from build123d import *

# Parameters (mm, degrees)
ESQUISSE2_R                                       = 76.2
ESQUISSE2_R_2                                     = 50.8
BOSS_EXTRU_1_DEPTH                                = 10
CHANFREIN1_SIZE                                   = 3
D_GAGEMENT_81_D                                   = 4.4958
FRAISAGE_POUR_VIS_T_TE_FRAIS_E_BOMB_E_D           = 5.1054
FRAISAGE_POUR_VIS_T_TE_FRAIS_E_BOMB_E_CSINK_D     = 9.779
FRAISAGE_POUR_VIS_T_TE_FRAIS_E_BOMB_E_CSINK_ANGLE = 82


with BuildPart() as part:
    # Esquisse2 → Boss.-Extru.1 (new body)
    with BuildSketch(Plane.XY):
        Circle(ESQUISSE2_R)
        Circle(ESQUISSE2_R_2, mode=Mode.SUBTRACT)
    extrude(amount=BOSS_EXTRU_1_DEPTH)

    # Chanfrein1
    chanfrein1_edges = [part.edges().sort_by_distance(p)[0] for p in [
        (-76.2, 0, 0),
    ]]
    chamfer(chanfrein1_edges, length=CHANFREIN1_SIZE)

    # Dégagement #81 (through all)
    with Locations(Plane(origin=(0, 0, 0), x_dir=(-1, 0, 0), z_dir=(0, 0, -1))):
        with Locations((0, 59.65), (51.658415336, 29.825), (29.825, 51.658415336), (59.65, 0), (51.658415336, -29.825), (29.825, -51.658415336), (0, -59.65), (-29.825, -51.658415336), (-51.658415336, -29.825), (-59.65, 0), (-51.658415336, 29.825), (-29.825, 51.658415336)):
            Hole(D_GAGEMENT_81_D / 2)

    # Fraisage pour vis à tête fraisée bombée #101 (through all)
    with Locations(Plane(origin=(0, 0, 0), x_dir=(-1, 0, 0), z_dir=(0, 0, -1))):
        with Locations((48.083261121, -48.083261121), (-65.682956188, -17.599695067), (17.599695067, 65.682956188)):
            CounterSinkHole(FRAISAGE_POUR_VIS_T_TE_FRAIS_E_BOMB_E_D / 2, FRAISAGE_POUR_VIS_T_TE_FRAIS_E_BOMB_E_CSINK_D / 2, counter_sink_angle=FRAISAGE_POUR_VIS_T_TE_FRAIS_E_BOMB_E_CSINK_ANGLE)


solid = part.part
The model under review builds one solid part; all positions refer to its coordinate system, in mm. Coordinates: 2 decimals unless noted, no trailing zeros. Write each loop counter-clockwise with the first axis right and the second up, starting at its lowest first coordinate (ties: lowest second). Pieces come first, ordered by that corner, then holes. Notation, with made-up numbers: (54.25, -6.5) - (87.25, -6.5) arc R23 cw to (87.25, 1.5) - close; hole circle Ø8 at (-38, 26). An arc over 180 degrees is marked (long way). Answer as CSV lines item,"result".
(1) Mouldability with a two-part tool opening along X and no side actions: class faces 1 (the conical face through (-45.62, -49.1, 2.56)), 2 (the flat face through (-52, 1, 10)), 3 (the conical face through (69.959, 22.031, 0.146)) as pulls with the +X half, pulls with the -X half, needs draft (parallel to the pull), parting line crosses it, or undercut.
Data:
face 1,"undercut"
face 2,"needs draft"
face 3,"parting line crosses it"
(2) Clearance check with flat-ended pins moving along their axes: pin 1 Ø1.5 at (x, z) = (7.5, 5) entering from -Y; pin 2 Ø4 at (y, z) = (36.5, 7.5) entering from -X; pin 3 Ø6 at (y, z) = (23.5, 5.5) entering from -X. State where each tip first meets the part, or that it passes through.
Data:
pin 1,"stops at y = -75.9"
pin 2,"stops at x = -67.94"
pin 3,"stops at x = -73.39"
(3) We need section A-A (y = 0). Give the boundary of the cut face in (x, z), plus the area to 3 significant figures.
Data:
outline,"(-76.2, 3) - (-73.2, 0) - (-61.9, 0) - (-61.9, 10) - (-76.2, 10) - close; (-57.4, 0) - (-50.8, 0) - (-50.8, 10) - (-57.4, 10) - close; (50.8, 0) - (57.4, 0) - (57.4, 10) - (50.8, 10) - close; (61.9, 0) - (73.2, 0) - (76.2, 3) - (76.2, 10) - (61.9, 10) - close"
area,"409 mm2"
(4) We need section C-C (z = 6.75). Count the separate pieces of the cut face and the enclosed holes in it, plus the area to 3 significant figures.
Data:
separate pieces,"1"
enclosed holes,"16"
area,"9,880 mm2"
(5) For line 1 along Y through (x, z) = (0, 6); line 2 along Y through (x, z) = (29, 6); line 3 along X through (y, z) = (11, 8.75), list the stretches that pass through material, from the lowest coordinate up. Write a range as [from, to].
Data:
line 1,"y = [-76.2, -61.9], [-57.4, -50.8], [50.8, 57.4], [61.9, 76.2]"
line 2,"y = [-70.47, -53.75], [-49.57, -41.71], [41.71, 49.57], [53.75, 70.47]"
line 3,"x = [-75.4, -49.59], [49.59, 75.4]"
